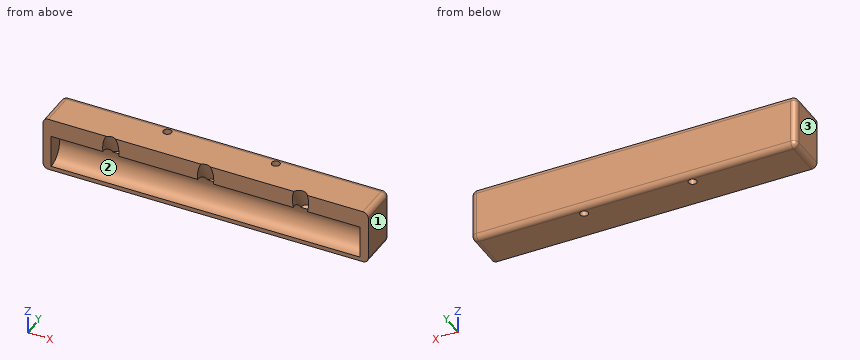
from build123d import *

# Parameters (mm, degrees)
SKETCH1_W           = 120
SKETCH1_H           = 15
BOSS_EXTRUDE1_DEPTH = 15
CUT_EXTRUDE4_START  = -3
SKETCH2_R           = 6
CUT_EXTRUDE4_DEPTH  = 114
SKETCH3_W           = 120
SKETCH3_H           = 15
BOSS_EXTRUDE2_DEPTH = 5
SKETCH5_R           = 3
CUT_EXTRUDE5_DEPTH  = 11
SKETCH6_R           = 1.5
CUT_EXTRUDE6_DEPTH  = 66
FILLET2_R           = 2
FILLET3_R           = 2
FILLET4_R           = 2
FILLET5_R           = 2


with BuildPart() as part:
    # Sketch1 → Boss-Extrude1 (new body)
    with BuildSketch(Plane(origin=(0, 0, 0), x_dir=(1, 0, 0), z_dir=(0, 1, 0))):
        Rectangle(SKETCH1_W, SKETCH1_H)
    extrude(amount=BOSS_EXTRUDE1_DEPTH)

    # Sketch2 → Cut-Extrude4 (cut)
    with BuildSketch(Plane.ZY.offset(60).offset(CUT_EXTRUDE4_START)):
        Circle(SKETCH2_R)
    extrude(amount=-CUT_EXTRUDE4_DEPTH, mode=Mode.SUBTRACT)

    # Sketch3 → Boss-Extrude2 (add)
    with BuildSketch(Plane.XY.offset(7.5)):
        with Locations((0, 7.5)):
            Rectangle(SKETCH3_W, SKETCH3_H)
    extrude(amount=BOSS_EXTRUDE2_DEPTH)

    # Sketch5 → Cut-Extrude5 (cut)
    with BuildSketch(Plane(origin=(0, -5.412658774, 9.375), x_dir=(1, 0, 0), z_dir=(0, -0.499999999999998, 0.8660254037844398))):
        with Locations((-35, 3.75)):
            Circle(SKETCH5_R)
        with Locations((0, 3.75)):
            Circle(SKETCH5_R)
        with Locations((35, 4.610408675)):
            Circle(SKETCH5_R)
    extrude(amount=-CUT_EXTRUDE5_DEPTH, mode=Mode.SUBTRACT)

    # Sketch6 → Cut-Extrude6 (cut, through all)
    with BuildSketch(Plane.XY.offset(12.5)):
        with Locations((-20, 11.5)):
            Circle(SKETCH6_R)
        with Locations((20, 11.5)):
            Circle(SKETCH6_R)
    extrude(amount=-CUT_EXTRUDE6_DEPTH, mode=Mode.SUBTRACT)

    # Fillet2
    fillet2_edges = [part.edges().sort_by_distance(p)[0] for p in [
        (0, 15, -7.5),
    ]]
    fillet(fillet2_edges, radius=FILLET2_R - 0.0001)  # a hair under: the kernel refuses the full size

    # Fillet3
    fillet3_edges = [part.edges().sort_by_distance(p)[0] for p in [
        (0, 15, 12.5),
    ]]
    fillet(fillet3_edges, radius=FILLET3_R - 0.0001)  # a hair under: the kernel refuses the full size

    # Fillet4
    fillet4_edges = [part.edges().sort_by_distance(p)[0] for p in [
        (-60, 6.50005, -7.5),
        (-60, 15, 2.5),
        (-60, 14.414242852, -6.914242852),
        (-60, 6.50005, 12.5),
        (-60, 14.414242852, 11.914242852),
    ]]
    fillet(fillet4_edges, radius=FILLET4_R - 0.0001)  # a hair under: the kernel refuses the full size

    # Fillet5
    fillet5_edges = [part.edges().sort_by_distance(p)[0] for p in [
        (60, 6.50005, 12.5),
        (60, 6.50005, -7.5),
        (60, 14.414242852, -6.914242852),
        (60, 15, 2.5),
        (60, 14.414242852, 11.914242852),
    ]]
    fillet(fillet5_edges, radius=FILLET5_R - 0.0001)  # a hair under: the kernel refuses the full size


solid = part.part
CAD build for the part. Positions are in the model's coordinates, mm. Face numbers are marked on the shaded views. Give positions to 0.01 mm unless a question says otherwise; leave off trailing zeros. Loops run counter-clockwise (first coordinate to the right, second up) from the corner with the lowest first, then second, coordinate; pieces in that order, holes last. Notation, with made-up numbers: M 69.25,14.5 L 105.25,14.5 A3 ccw 105.25,19.5 Z; hole C 50,84 d1. An arc over 180 degrees is marked long. Write each question's results on one line, items separated by ' | '.
Q1. Band-saw the part on C-C on z = 0. Write the cut outline in (x, y), and give its area (3 significant figures).
Geometry check:
outline: M -60,0 L -57,0 L -57,6 L 57,6 L 57,0 L 60,0 L 60,13 A2 ccw 58,15 L -58,15 A2 ccw -60,13 Z; hole C -20,11.5 d3; hole C 20,11.5 d3 | area: 1,100 mm²
Q2. Band-saw the part on B-B on y = 11.5. Write the cut outline in (x, z).
Geometry check:
outline: M -60,-5.5 A2 ccw -58,-7.5 L -21.5,-7.5 L -21.5,12.5 L -58,12.5 A2 ccw -60,10.5 Z; M -18.5,-7.5 L 18.5,-7.5 L 18.5,12.5 L -18.5,12.5 Z; M 21.5,-7.5 L 58,-7.5 A2 ccw 60,-5.5 L 60,10.5 A2 ccw 58,12.5 L 21.5,12.5 Z
Q3. Probe probe 1 along Y at (x, z) = (20, 7); probe 2 along X at (y, z) = (2.5, 7); probe 3 along X at (y, z) = (12.5, -5). List the from-to ranges inside material, lowest first.
Geometry check:
probe 1: y = 0 to 10, 13 to 15 | probe 2: x = -60 to -37.31, -32.69 to -2.31, 2.31 to 32.19, 37.81 to 60 | probe 3: x = -60 to -21.12, -18.88 to 18.88, 21.12 to 60
Q4. Flat gauge pin, fed straight in: P1, Ø1, axis at x = 2, z = -5, coming from the -Y side. Where does the tip first touch, or does it go through?
Geometry check:
P1: stops at y = 2.4
Q5. Mould opens along X. For the marked faces 1, 2 and 3 say: pulls with the +X half, pulls with the -X half, needs draft (parallel to the pull), parting line crosses it, or undercut.
Geometry check:
face 1: pulls with the +X half | face 2: undercut | face 3: pulls with the -X half
